Source: CAD feature listing. Evaluate the final solid. Frame: model axes, mm. A direction names the side the tool comes from. Round coordinates to 2 decimals unless told otherwise and drop trailing zeros. Order: outer loops, then holes, each group sorted by start corner. A loop starts at its lowest first (then second) coordinate and runs counter-clockwise, first axis right, second up. Notation, with made-up numbers: (48, -7) - (84, -7) arc R28 ccw to (84, 12) - close; hole circle Ø8 at (40.5, -3.75). An arc over 180 degrees is marked (long way). Put each result on its own line as item: value. Start each with the question number.
1) Section A-A on z = -71.5. Output: boundary loops of the cut face in (x, y).
2) Access query for faces 1 (the face through (55.2, -7.51, -84.46)), 2 (the face through (-1, -15.24, -11)). Directions: +Z, -Z, +X, -X, +Y, -Y. A direction counts if a zero-diameter tool reaches every point of the face in a straight line with its end or side. Return the directions, or none.
3) Section C-C on x = 0. Output: boundary loops of the cut face in (y, z).
4) Mould query, pull axis X, two halves, no side actions, for faces 3 (the face through (-76.2, -8, -50)), 4 (the face through (-55.78, -7.51, -84.93)), 5 (the face through (-1, 0, -11)). Classes: +X half, -X half, draft (parallel to the pull), parting line (faces both ways), or undercut.
5) Line query: probe 1 along Z at (x, y) = (-2, -13); probe 2 along X at (y, z) = (-14.5, -89.5); probe 3 along X at (y, z) = (-8, -78.5). Output: solid intervals per line, ascending. Write a range as [from, to].
6) Section B-B on y = -6. Output: boundary loops of the cut face in (x, z), then the cut area to 3 significant figures.
7) Contact query for flat-ended pins moving along their axis: P1, Ø3, axis at x = -58.5, y = -4, coming from the +Z side; P2, Ø8, axis at x = -15, y = -6.5, coming from the +Z side; P3, Ø3, axis at y = -7.5, z = 54, coming from the -X side. Output: stop coordinate, or through.
```python
from build123d import *

# Parameters (mm, degrees)
F1_DEPTH = 15.24


# Not quite as in the source:
# - a feature names something its author has since deleted; it is built from what else it names


with BuildPart() as f1:
    # F0 (on Front) → F1 (new body)
    with BuildSketch(Plane.XZ):
        with BuildLine():
            ThreePointArc((34.7869106265, -67.7960975946), (65.0276963676, -39.7220178884), (76.2, 0))
            ThreePointArc((76.2, 0), (0, 76.2), (-76.2, 0))
            ThreePointArc((-76.2, 0), (-65.0276963676, -39.7220178884), (-34.7869106265, -67.7960975946))
            ThreePointArc((-34.7869106265, -67.7960975946), (0, -76.2), (34.7869106265, -67.7960975946))
        make_face()
        with BuildLine():
            Line((76.2, -101.6), (76.2, 0))
            ThreePointArc((76.2, 0), (65.0276963676, -39.7220178884), (34.7869106265, -67.7960975946))
            Line((34.7869106265, -67.7960975946), (76.2, -101.6))
        make_face()
        with BuildLine():
            ThreePointArc((-34.7869106265, -67.7960975946), (-65.0276963676, -39.7220178884), (-76.2, 0))
            Line((-76.2, 0), (-76.2, -101.6))
            Line((-76.2, -101.6), (-34.7869106265, -67.7960975946))
        make_face()
    extrude(amount=F1_DEPTH)


solid = f1.part
```
Answer sheet:
1. outline: (-76.2, -15.24) - (-39.32, -15.24) - (-39.32, 0) - (-76.2, 0) - close; (-26.35, -15.24) - (26.35, -15.24) - (26.35, 0) - (-26.35, 0) - close; (39.32, -15.24) - (76.2, -15.24) - (76.2, 0) - (39.32, 0) - close
2. face 1: -Z, +Y, -Y
2. face 2: +Z, -Z, +X, -X, -Y
3. outline: (-15.24, -76.2) - (0, -76.2) - (0, 76.2) - (-15.24, 76.2) - close
4. face 3: -X half
4. face 4: undercut
4. face 5: draft
5. probe 1: [-76.17, 76.17]
5. probe 2: [-76.2, -61.38], [61.38, 76.2]
5. probe 3: [-76.2, -47.9], [47.9, 76.2]
6. outline: (-76.2, -101.6) - (-34.79, -67.8) arc R76.2 ccw to (34.79, -67.8) - (76.2, -101.6) - (76.2, 0) arc R76.2 ccw to (-76.2, 0) - close
6. area: 21,200 mm^2
7. P1: z = 50.57
7. P2: z = 75.4
7. P3: x = -55.23
